```python
from build123d import *

# Parameters (mm, degrees)
SKETCH1_W               = 75
SKETCH1_H               = 25
BOSS_EXTRUDE1_DEPTH     = 8
SKETCH5_W               = 25
SKETCH5_H               = 21
BOSS_EXTRUDE2_DEPTH     = 50
SKETCH7_W               = 16.7
SKETCH7_H               = 16.7
CUT_EXTRUDE3_DEPTH      = 45
SKETCH4_R               = 2.38125
CUT_EXTRUDE2_DEPTH      = 50.025503567
CUT_EXTRUDE1_DEPTH      = 45.760473635
CUT_EXTRUDE1_DEPTH_BACK = 5
SKETCH3_R               = 4
FILLET1_R               = 3


with BuildPart() as part:
    # Sketch1 → Boss-Extrude1 (new body)
    with BuildSketch(Plane(origin=(0, 0, 0), x_dir=(1, 0, 0), z_dir=(0, 1, 0))):
        Rectangle(SKETCH1_W, SKETCH1_H)
    extrude(amount=BOSS_EXTRUDE1_DEPTH)

    # Sketch5 → Boss-Extrude2 (add)
    with BuildSketch(Plane.ZY.offset(37.5)):
        with Locations((0, 18.5)):
            Rectangle(SKETCH5_W, SKETCH5_H)
    extrude(amount=-BOSS_EXTRUDE2_DEPTH)

    # Sketch7 → Cut-Extrude3 (cut)
    with BuildSketch(Plane(origin=(12.5, 0, 0), x_dir=(0, 0, -1), z_dir=(1, 0, 0))):
        with Locations((0, 16.35)):
            Rectangle(SKETCH7_W, SKETCH7_H)
    extrude(amount=-CUT_EXTRUDE3_DEPTH, mode=Mode.SUBTRACT)

    # Sketch4 → Cut-Extrude2 (cut, through all)
    with BuildSketch(Plane(origin=(0, 0, 0), x_dir=(1, 0, 0), z_dir=(0, 1, 0))):
        with Locations(Location((0, 0, 0), (0, 0, 90))):
            Circle(SKETCH4_R)
        with Locations(Location((25.4, 0, 0), (0, 0, 90))):
            Circle(SKETCH4_R)
        with Locations(Location((-25.4, 0, 0), (0, 0, 90))):
            Circle(SKETCH4_R)
    extrude(amount=CUT_EXTRUDE2_DEPTH, mode=Mode.SUBTRACT)

    # Sketch3 → Cut-Extrude1 (cut, two sides: drawn at the far end of the back side and taken through both)
    with BuildSketch(Plane(origin=(0, 8, 0), x_dir=(1, 0, 0), z_dir=(0, 1, 0)).offset(-CUT_EXTRUDE1_DEPTH_BACK)):
        with Locations(Location((0, 0, 0), (0, 0, 90))):
            Circle(SKETCH3_R)
        with Locations(Location((25.4, 0, 0), (0, 0, 90))):
            Circle(SKETCH3_R)
        with Locations(Location((-25.4, 0, 0), (0, 0, 90))):
            Circle(SKETCH3_R)
    extrude(amount=CUT_EXTRUDE1_DEPTH + CUT_EXTRUDE1_DEPTH_BACK, mode=Mode.SUBTRACT)

    # Fillet1
    fillet1_edges = [part.edges().sort_by_distance(p)[0] for p in [
        (25, 8, 12.5),
        (12.5, 18.5, -12.5),
        (12.5, 29, 0),
        (-12.5, 29, -12.5),
        (12.5, 18.5, 12.5),
        (-12.5, 29, 12.5),
        (12.5, 8, -10.425),
        (-37.5, 29, 0),
        (12.5, 8, 10.425),
        (37.5, 8, 0),
        (37.5, 4, 12.5),
        (-37.5, 14.5, 12.5),
        (-37.5, 14.5, -12.5),
        (37.5, 4, -12.5),
        (25, 8, -12.5),
    ]]
    fillet(fillet1_edges, radius=FILLET1_R)


solid = part.part
```
The model under review builds one solid part; all positions refer to its coordinate system, in mm. A direction names the side the tool comes from. Give positions to 0.01 mm unless a question says otherwise; leave off trailing zeros. Write each loop counter-clockwise with the first axis right and the second up, starting at its lowest first coordinate (ties: lowest second). Pieces come first, ordered by that corner, then holes. Notation, with made-up numbers: (58.25, -30.75) -> (91.25, -30.75) arc R7 ccw to (91.25, -21.75) -> close; hole circle Ø8 at (33, 37). An arc over 180 degrees is marked (long way). Answer in a Markdown table with one row per item.
1) Add section C-C on x = 6. State the section outline as (y, z) points.
Worked answers:
| item | result |
|---|---|
| outline | (0, -12.5) -> (26, -12.5) arc R3 ccw to (29, -9.5) -> (29, 9.5) arc R3 ccw to (26, 12.5) -> (0, 12.5) -> close; hole (8, -8.35) -> (24.7, -8.35) -> (24.7, 8.35) -> (8, 8.35) -> close |
2) For L1, parallel to X at y = 2.25, z = 0; L2, parallel to Z at x = -25.4, y = 7; L3, parallel to X at y = 6, z = -3, list the stretches that pass through material, from the lowest coordinate up. Write a range as [from, to].
Worked answers:
| item | result |
|---|---|
| L1 | [-37.5, -27.78], [-23.02, -2.38], [2.38, 23.02], [27.78, 37.5] |
| L2 | [-12.5, -4], [4, 12.5] |
| L3 | [-37.5, -28.05], [-22.75, -2.65], [2.65, 22.75], [28.05, 37.33] |
3) Mouldability with a two-part tool opening along X and no side actions: class faces 1 (the cylindrical face through (-21.495, 5.465, 0.867)), 2 (the flat face through (-8, 13, 12.5)), 3 (the cylindrical face through (11.6, 18.6, -11.64)) as +X half, -X half, draft (parallel to the pull), parting line (faces both ways), or undercut.
Worked answers:
| item | result |
|---|---|
| face 1 | undercut |
| face 2 | draft |
| face 3 | +X half |
4) Add section B-B on y = 2. State the section outline as (x, z) points, plus the area to 3 significant figures.
Worked answers:
| item | result |
|---|---|
| outline | (-37.5, -9.5) arc R3 ccw to (-34.5, -12.5) -> (34.5, -12.5) arc R3 ccw to (37.5, -9.5) -> (37.5, 9.5) arc R3 ccw to (34.5, 12.5) -> (-34.5, 12.5) arc R3 ccw to (-37.5, 9.5) -> close; hole circle Ø4.76 at (-25.4, 0); hole circle Ø4.76 at (0, 0); hole circle Ø4.76 at (25.4, 0) |
| area | 1,810 mm² |
5) Tool access review of faces 4 (the cylindrical face through (29.305, 5.465, 0.867)), 5 (the flat face through (-10, 24.7, 0)), 6 (the cylindrical face through (36.64, 2.54, 11.6)), 7 (the cylindrical face through (36.64, 7.1, -0.13)), 8 (the cylindrical face through (11.64, 18.6, 11.6)): name each direction out of +Z, -Z, +X, -X, +Y, -Y from which nothing blocks a thin tool from reaching the whole face with its end or side.
Worked answers:
| item | result |
|---|---|
| face 4 | +Y |
| face 5 | +X |
| face 6 | +Z, +X, +Y, -Y |
| face 7 | +Z, -Z, +X, +Y |
| face 8 | +Z, +X, +Y |
6) Add section A-A on x = 25.4. State the section outline as (y, z) points, plus the area to 3 significant figures.
Worked answers:
| item | result |
|---|---|
| outline | (0, -12.5) -> (5, -12.5) arc R3 ccw to (8, -9.5) -> (8, -4) -> (3, -4) -> (3, -2.38) -> (0, -2.38) -> close; (0, 2.38) -> (3, 2.38) -> (3, 4) -> (8, 4) -> (8, 9.5) arc R3 ccw to (5, 12.5) -> (0, 12.5) -> close |
| area | 142 mm² |
7) Add section D-D on z = 0. Count the separate pieces of the cut face and the enclosed holes in it, plus the area to 3 significant figures.
Worked answers:
| item | result |
|---|---|
| separate pieces | 6 |
| enclosed holes | 0 |
| area | 661 mm² |
8) Clearance check with flat-ended pins moving along their axes: P1, Ø7, axis at x = 0, z = 0, coming from the -Y side; P2, Ø6.5, axis at x = 25.4, z = 0, coming from the +Y side; P3, Ø9, axis at x = 24.5, z = -2, coming from the +Y side; P4, Ø4.5, axis at y = 16.5, z = -3.5, coming from the +X side. State where each tip first meets the part, or that it passes through.
Worked answers:
| item | result |
|---|---|
| P1 | y = 0 |
| P2 | y = 3 |
| P3 | y = 8 |
| P4 | x = -32.5 |
